Geometry: final body of the model. Coordinates: model frame, mm. A direction names the side the tool comes from. Give positions to 0.01 mm unless a question says otherwise; leave off trailing zeros. Write each loop counter-clockwise with the first axis right and the second up, starting at its lowest first coordinate (ties: lowest second). Pieces come first, ordered by that corner, then holes. Notation, with made-up numbers: M 26.25,0.5 L 84.25,0.5 A22 ccw 84.25,11.5 Z; hole C 28,-30 d2. An arc over 180 degrees is marked long. Answer as a JSON object with one key per item and string values.
from build123d import *

# Parameters (mm, degrees)
BOX001_W         = 20
BOX001_H         = 590
BOX001_DEPTH     = 20
ARRAY001_X_COUNT = 2
ARRAY001_X_PITCH = 690
ARRAY001_Z_COUNT = 2
ARRAY001_Z_PITCH = 80
BOX003_W         = 20
BOX003_H         = 590
BOX003_DEPTH     = 20
ARRAY002_X_COUNT = 2
ARRAY002_X_PITCH = 690
ARRAY002_Z_COUNT = 2
ARRAY002_Z_PITCH = 90
BOX002_W         = 670
BOX002_H         = 20
BOX002_DEPTH     = 20
ARRAY003_Y_COUNT = 2
ARRAY003_Y_PITCH = 610
ARRAY003_Z_COUNT = 2
ARRAY003_Z_PITCH = 80
BOX004_W         = 670
BOX004_H         = 20
BOX004_DEPTH     = 20
ARRAY004_Y_COUNT = 2
ARRAY004_Y_PITCH = 610
ARRAY004_Z_COUNT = 2
ARRAY004_Z_PITCH = 90
BOX_W            = 20
BOX_H            = 20
BOX_DEPTH        = 700
ARRAY_X_COUNT    = 2
ARRAY_X_PITCH    = 690
ARRAY_Y_COUNT    = 2
ARRAY_Y_PITCH    = 610


with BuildPart() as laterales_inferiores:
    # Box001 → Box001 (new body)
    with BuildSketch(Plane(origin=(0, 20, 0), x_dir=(1, 0, 0), z_dir=(0, 0, 1))):
        with Locations((10, 295)):
            Rectangle(BOX001_W, BOX001_H)
    extrude(amount=BOX001_DEPTH)

    # Array001 X: Laterales inferiores ×2


with BuildPart() as laterales_inferiores_1:
    add(laterales_inferiores.part)
    with Locations(*[(i * ARRAY001_X_PITCH, 0, 0) for i in range(1, ARRAY001_X_COUNT)]):
        add(laterales_inferiores.part)

    # Array001 Z: Laterales inferiores ×2


with BuildPart() as laterales_inferiores_2:
    add(laterales_inferiores_1.part)
    with Locations(*[(0, 0, i * ARRAY001_Z_PITCH) for i in range(1, ARRAY001_Z_COUNT)]):
        add(laterales_inferiores_1.part)


with BuildPart() as laterales_superiores:
    # Box003 → Box003 (new body)
    with BuildSketch(Plane(origin=(0, 20, 0), x_dir=(1, 0, 0), z_dir=(0, 0, 1))):
        with Locations((10, 295)):
            Rectangle(BOX003_W, BOX003_H)
    extrude(amount=BOX003_DEPTH)

    # Array002 X: Laterales Superiores ×2


with BuildPart() as laterales_superiores_1:
    add(laterales_superiores.part)
    with Locations(*[(i * ARRAY002_X_PITCH, 0, 0) for i in range(1, ARRAY002_X_COUNT)]):
        add(laterales_superiores.part)

    # Array002 Z: Laterales Superiores ×2


with BuildPart() as laterales_superiores_2:
    add(laterales_superiores_1.part)
    with Locations(*[(0, 0, i * ARRAY002_Z_PITCH) for i in range(1, ARRAY002_Z_COUNT)]):
        add(laterales_superiores_1.part)


with BuildPart() as laterales_superiores_3:
    # Array002 placement: moved
    add(laterales_superiores_2.part.moved(Location((0, 0, 590))))


with BuildPart() as frontales_inferiores:
    # Box002 → Box002 (new body)
    with BuildSketch(Plane(origin=(20, 0, 0), x_dir=(1, 0, 0), z_dir=(0, 0, 1))):
        with Locations((335, 10)):
            Rectangle(BOX002_W, BOX002_H)
    extrude(amount=BOX002_DEPTH)

    # Array003 Y: Frontales inferiores ×2


with BuildPart() as frontales_inferiores_1:
    add(frontales_inferiores.part)
    with Locations(*[(0, i * ARRAY003_Y_PITCH, 0) for i in range(1, ARRAY003_Y_COUNT)]):
        add(frontales_inferiores.part)

    # Array003 Z: Frontales inferiores ×2


with BuildPart() as frontales_inferiores_2:
    add(frontales_inferiores_1.part)
    with Locations(*[(0, 0, i * ARRAY003_Z_PITCH) for i in range(1, ARRAY003_Z_COUNT)]):
        add(frontales_inferiores_1.part)


with BuildPart() as frontales_superiores:
    # Box004 → Box004 (new body)
    with BuildSketch(Plane(origin=(20, 0, 0), x_dir=(1, 0, 0), z_dir=(0, 0, 1))):
        with Locations((335, 10)):
            Rectangle(BOX004_W, BOX004_H)
    extrude(amount=BOX004_DEPTH)

    # Array004 Y: Frontales superiores ×2


with BuildPart() as frontales_superiores_1:
    add(frontales_superiores.part)
    with Locations(*[(0, i * ARRAY004_Y_PITCH, 0) for i in range(1, ARRAY004_Y_COUNT)]):
        add(frontales_superiores.part)

    # Array004 Z: Frontales superiores ×2


with BuildPart() as frontales_superiores_2:
    add(frontales_superiores_1.part)
    with Locations(*[(0, 0, i * ARRAY004_Z_PITCH) for i in range(1, ARRAY004_Z_COUNT)]):
        add(frontales_superiores_1.part)


with BuildPart() as frontales_superiores_3:
    # Array004 placement: moved
    add(frontales_superiores_2.part.moved(Location((0, 0, 590))))


with BuildPart() as obj1:
    # Box → Box (new body)
    with BuildSketch(Plane.XY):
        with Locations((10, 10)):
            Rectangle(BOX_W, BOX_H)
    extrude(amount=BOX_DEPTH)

    # Array X: obj1_2


with BuildPart() as obj1_1:
    add(obj1.part)
    with Locations(*[(i * ARRAY_X_PITCH, 0, 0) for i in range(1, ARRAY_X_COUNT)]):
        add(obj1.part)

    # Array Y: obj1_2


with BuildPart() as obj1_2:
    add(obj1_1.part)
    with Locations(*[(0, i * ARRAY_Y_PITCH, 0) for i in range(1, ARRAY_Y_COUNT)]):
        add(obj1_1.part)

    # Fusion: union Laterales inferiores, Laterales Superiores, Frontales inferiores, Frontales superiores
    add(laterales_inferiores_2.part)
    add(laterales_superiores_3.part)
    add(frontales_inferiores_2.part)
    add(frontales_superiores_3.part)


solid = obj1_2.part
1) Pull-direction query (Y, two-part tool) for faces 1 (the flat face through (327, 630, 608)), 2 (the flat face through (350, 10, 80)), 3 (the flat face through (10, 319, 610)); classes: pulls with the +Y half, pulls with the -Y half, needs draft (parallel to the pull), parting line crosses it, or undercut.
Geometry check:
{"face 1": "pulls with the +Y half", "face 2": "needs draft", "face 3": "undercut"}
2) Cut plane A-A on x = 529. Give the number of separate pieces and of enclosed holes in the cut face, and give its area (3 significant figures).
Geometry check:
{"separate pieces": "8", "enclosed holes": "0", "area": "3,200 mm2"}
3) Set-up query: faces 4 (the flat face through (327, 13, 700)), 5 (the flat face through (350, 10, 100)), 6 (the flat face through (690, 311, 10)), 7 (the flat face through (700, 610, 342)). Return all of +Z, -Z, +X, -X, +Y, -Y with unobstructed straight access to the full face (end or side cutting, diameter ignored); none if empty.
Geometry check:
{"face 4": "+Z, +X, -X, +Y, -Y", "face 5": "+Y, -Y", "face 6": "+Z, -Z", "face 7": "+X, -X"}
4) Line query: line 1 (Y direction, x = 502, z = 99.5). Output: solid intervals per line, ascending. Write a range as from..to.
Geometry check:
{"line 1": "y = 0..20, 610..630"}
5) Cut plane B-B on z = 457.5. Return loops of the section in (x, y), and give its area (3 significant figures).
Geometry check:
{"outline": "M 0,0 L 20,0 L 20,20 L 0,20 Z; M 0,610 L 20,610 L 20,630 L 0,630 Z; M 690,0 L 710,0 L 710,20 L 690,20 Z; M 690,610 L 710,610 L 710,630 L 690,630 Z", "area": "1,600 mm2"}
